```python
from build123d import *

# Parameters (mm, degrees)
STOCK_HAMMERSAW_START                 = -4.7625
STOCK_HAMMERSAW_MULTIBODY_1_OUTLINE_R = 3.175
STOCK_HAMMERSAW_MULTIBODY_1_DEPTH     = 9.525
BOSS_EXTRUDE3_DEPTH                   = 9.525


# Read off the part's stored shape, not the designer's step: Stock-HammerSaw Multibody-1
with BuildPart() as part:
    # Stock-HammerSaw Multibody-1 outline → Stock-HammerSaw Multibody-1 (new body)
    with BuildSketch(Plane.YZ.offset(STOCK_HAMMERSAW_START)):
        with BuildLine():
            ThreePointArc((14.114185067, -169.917610968), (5.877809274, -169.350270146), (1.524707151, -176.365272906))
            Line((1.524707151, -176.365272906), (1.27, -195.521646474))
            Line((1.27, -195.521646474), (13.572128535, -195.521646474))
            Line((13.572128535, -195.521646474), (13.572128535, -194.202498844))
            Line((13.572128535, -194.202498844), (12.230315554, -191.32497162))
            ThreePointArc((12.230315554, -191.32497162), (14.283881996, -181.92450591), (23.892574452, -181.415664109))
            Line((23.892574452, -181.415664109), (26.077900674, -178.294694821))
            Line((26.077900674, -178.294694821), (14.114185067, -169.917610968))
        make_face()
        with Locations((9.525, -176.471646474)):
            Circle(STOCK_HAMMERSAW_MULTIBODY_1_OUTLINE_R, mode=Mode.SUBTRACT)
    extrude(amount=STOCK_HAMMERSAW_MULTIBODY_1_DEPTH)

    # Sketch3 → Boss-Extrude3 (add)
    with BuildSketch(Plane(origin=(4.7625, 0, 0), x_dir=(0, 0, -1), z_dir=(1, 0, 0))):
        Polygon((195.521646474, 13.572128535), (227.271646474, 6.35), (227.271646474, 9.525), (252.671646474, 0), (227.271646474, 0), (195.521646474, 1.27), align=None)
    extrude(amount=-BOSS_EXTRUDE3_DEPTH)


solid = part.part
```
The model under review builds one solid part; all positions refer to its coordinate system, in mm. A direction names the side the tool comes from. Give positions to 0.01 mm unless a question says otherwise; leave off trailing zeros. Write each loop counter-clockwise with the first axis right and the second up, starting at its lowest first coordinate (ties: lowest second). Pieces come first, ordered by that corner, then holes. Notation, with made-up numbers: (36.25, -8.5) - (43.25, -8.5) arc R11 cw to (43.25, -0.5) - close; hole circle Ø2 at (37, 75.25). An arc over 180 degrees is marked (long way). Answer in a Markdown table with one row per item. Add a question column.
1. Insertion check: P1, Ø4, axis at x = -1, z = -217.5, coming from the -Y side; P2, Ø2.5, axis at x = 2.5, y = 8, coming from the +Z side; P3, Ø1.5, axis at x = -0.5, z = -202.5, coming from the +Y side. Each pin has a flat end and moves straight along its axis. Give the tip position at first contact, or say it passes through.
2. We need section D-D on z = -235. Write out the cut boundary in (x, y), then the cut area to 3 significant figures.
3. Wall thickness on line 1 along Y through (x, z) = (2.25, -175.5); line 2 along Y through (x, z) = (1.5, -174); line 3 along Y through (x, z) = (-1, -194): over which ranges is each line inside the solid? List them lowest first. Write a range as [from, to].
4. We need section C-C on y = 21.75. Write out the cut boundary in (x, z).
5. Tool access review of faces 1 (the flat face through (-0.07, 12.91, -192.78)), 2 (the flat face through (0.07, 4.83, -239.79)): name each direction out of +Z, -Z, +X, -X, +Y, -Y from which nothing blocks a thin tool from reaching the whole face with its end or side.
6. We need section B-B on y = 7.5. Write out the cut boundary in (x, z).
7. Draft analysis for pull direction Z (two halves, no side actions). For faces 3 (the flat face through (-4.762, 8, -201)), 4 (the cylindrical face through (-0.07, 10.99, -179.29)), 5 (the flat face through (0.067, 0.626, -211.619)), 6 (the flat face through (-0.07, 24.97, -179.88)), state which applies: +Z half, -Z half, draft (parallel to the pull), parting line (faces both ways), or undercut.
Ans:
| question | item | result |
|---|---|---|
| 1 | P1 | stops at y = 0.31 |
| 1 | P2 | stops at z = -168.48 |
| 1 | P3 | stops at y = 12.16 |
| 2 | outline | (-4.76, 0) - (4.76, 0) - (4.76, 6.63) - (-4.76, 6.63) - close |
| 2 | area | 63.1 mm^2 |
| 3 | line 1 | y = [1.58, 6.5], [12.55, 22.09] |
| 3 | line 2 | y = [1.92, 7.53], [11.52, 19.94] |
| 3 | line 3 | y = [1.29, 13.48] |
| 4 | outline | (-4.76, -180.39) - (4.76, -180.39) - (4.76, -175.26) - (-4.76, -175.26) - close |
| 5 | face 1 | +X, -X, +Y |
| 5 | face 2 | -Z, +X, -X, +Y |
| 6 | outline | (-4.76, -232.67) - (4.76, -232.67) - (4.76, -227.27) - (-4.76, -227.27) - close; (-4.76, -222.22) - (4.76, -222.22) - (4.76, -178.92) - (-4.76, -178.92) - close; (-4.76, -174.03) - (4.76, -174.03) - (4.76, -168.73) - (-4.76, -168.73) - close |
| 7 | face 3 | draft |
| 7 | face 4 | undercut |
| 7 | face 5 | +Z half |
| 7 | face 6 | -Z half |
